Part model, mm, in its own coordinate system. A direction names the side the tool comes from. Give positions to 0.01 mm unless a question says otherwise; leave off trailing zeros. Order: outer loops, then holes, each group sorted by start corner. A loop starts at its lowest first (then second) coordinate and runs counter-clockwise, first axis right, second up. Notation, with made-up numbers: (-13.75, -32) - (16.25, -32) arc R22 ccw to (16.25, 1) - close; hole circle Ø3 at (-16.75, 9). An arc over 180 degrees is marked (long way). One line per item, written item: value.
```python
from build123d import *

# Parameters (mm, degrees)
MODEL_R                 = 1.7
MODEL_R_2               = 1.600279216
SALIENTE_EXTRUIR1_DEPTH = 3


with BuildPart() as part:
    # Model → Saliente-Extruir1 (new body)
    with BuildSketch(Plane.XY):
        with BuildLine():
            Line((74.679802956, 300.758040435), (5.677398721, 300.758040435))
            ThreePointArc((5.677398721, 300.758040435), (4.61673855, 300.318700606), (4.177398721, 299.258040435))
            Line((4.177398721, 299.258040435), (4.177398721, 221.253430577))
            ThreePointArc((4.177398721, 221.253430577), (4.61673855, 220.192770405), (5.677398721, 219.753430577))
            Line((5.677398721, 219.753430577), (28.17721751, 219.753430577))
            ThreePointArc((28.17721751, 219.753430577), (28.884324291, 220.046323796), (29.17721751, 220.753430577))
            Line((29.17721751, 220.753430577), (29.17721751, 227.730037779))
            ThreePointArc((29.17721751, 227.730037779), (28.884324291, 228.43714456), (28.17721751, 228.730037779))
            Line((28.17721751, 228.730037779), (7.17721751, 228.730037779))
            ThreePointArc((7.17721751, 228.730037779), (6.470110728, 229.022930998), (6.17721751, 229.730037779))
            Line((6.17721751, 229.730037779), (6.17721751, 291.370238846))
            ThreePointArc((6.17721751, 291.370238846), (6.470110728, 292.077345627), (7.17721751, 292.370238846))
            Line((7.17721751, 292.370238846), (19.67721751, 292.370238846))
            ThreePointArc((19.67721751, 292.370238846), (20.384324291, 292.663132064), (20.67721751, 293.370238846))
            Line((20.67721751, 293.370238846), (20.67721751, 298.097066693))
            ThreePointArc((20.67721751, 298.097066693), (20.970110728, 298.804173474), (21.67721751, 299.097066693))
            Line((21.67721751, 299.097066693), (58.179621744, 299.097066693))
            ThreePointArc((58.179621744, 299.097066693), (58.886728525, 298.804173474), (59.179621744, 298.097066693))
            Line((59.179621744, 298.097066693), (59.179621744, 294.260238845))
            ThreePointArc((59.179621744, 294.260238845), (59.472514963, 293.553132064), (60.179621744, 293.260238845))
            Line((60.179621744, 293.260238845), (73.179621744, 293.260238845))
            ThreePointArc((73.179621744, 293.260238845), (73.886728525, 292.967345627), (74.179621744, 292.260238845))
            Line((74.179621744, 292.260238845), (74.179621744, 227.755628988))
            ThreePointArc((74.179621744, 227.755628988), (73.886728525, 227.048522207), (73.179621744, 226.755628988))
            Line((73.179621744, 226.755628988), (56.179621744, 226.755628988))
            ThreePointArc((56.179621744, 226.755628988), (55.472514963, 226.462735769), (55.179621744, 225.755628988))
            Line((55.179621744, 225.755628988), (55.179621744, 220.753430577))
            ThreePointArc((55.179621744, 220.753430577), (55.472514963, 220.046323796), (56.179621744, 219.753430577))
            Line((56.179621744, 219.753430577), (74.679802956, 219.753430577))
            ThreePointArc((74.679802956, 219.753430577), (75.740463127, 220.192770405), (76.179802956, 221.253430577))
            Line((76.179802956, 221.253430577), (76.179802956, 299.258040435))
            ThreePointArc((76.179802956, 299.258040435), (75.740463127, 300.318700606), (74.679802956, 300.758040435))
        make_face()
        with Locations((17.676729717, 224.253096075)):
            Circle(MODEL_R, mode=Mode.SUBTRACT)
        with Locations((62.680137458, 224.253096075)):
            Circle(MODEL_R, mode=Mode.SUBTRACT)
        with Locations((8.677064219, 224.253096075)):
            Circle(MODEL_R_2, mode=Mode.SUBTRACT)
        with Locations((71.679802956, 224.253096075)):
            Circle(MODEL_R_2, mode=Mode.SUBTRACT)
        with Locations((17.676729717, 296.258040435)):
            Circle(MODEL_R, mode=Mode.SUBTRACT)
        with Locations((62.680137458, 296.258040435)):
            Circle(MODEL_R, mode=Mode.SUBTRACT)
        with Locations((71.679802956, 296.258040435)):
            Circle(MODEL_R_2, mode=Mode.SUBTRACT)
        with Locations((8.677064219, 296.258040435)):
            Circle(MODEL_R_2, mode=Mode.SUBTRACT)
    extrude(amount=SALIENTE_EXTRUIR1_DEPTH)


solid = part.part
```
1) Which spindle directions (+Z, -Z, +X, -X, +Y, -Y) get a long thin tool onto all of the face, cutting with end or side? Do faces 1 (the face through (18, 228.73, 1)), 2 (the face through (76.18, 260, 1)), 3 (the face through (55.18, 223, 1)). Say none if no direction does.
Answer:
face 1: +Z, -Z
face 2: +Z, -Z, +X, +Y, -Y
face 3: +Z, -Z, -Y
2) Slice it at A-A on x = 67.5. Write the cut outline in (y, z).
Answer:
outline: (219.75, 0) - (226.76, 0) - (226.76, 3) - (219.75, 3) - close; (293.26, 0) - (300.76, 0) - (300.76, 3) - (293.26, 3) - close
3) Slice it at C-C on x = 35. Write the cut outline in (y, z).
Answer:
outline: (299.1, 0) - (300.76, 0) - (300.76, 3) - (299.1, 3) - close
4) Slice it at B-B on y = 271. Write the cut outline in (x, z), then the cut area to 3 significant figures.
Answer:
outline: (4.18, 0) - (6.18, 0) - (6.18, 3) - (4.18, 3) - close; (74.18, 0) - (76.18, 0) - (76.18, 3) - (74.18, 3) - close
area: 12.0 mm2
5) Wall check: line 1 along X through (y, z) = (224.5, 1.15); line 2 along X through (y, z) = (270, 0.2); line 3 along Y through (x, z) = (26, 2.4). Give the ranges that are in metal, low to high. Write a range as [from, to].
Answer:
line 1: x = [4.18, 7.1], [10.26, 15.99], [19.36, 29.18], [55.18, 61], [64.36, 70.1], [73.26, 76.18]
line 2: x = [4.18, 6.18], [74.18, 76.18]
line 3: y = [219.75, 228.73], [299.1, 300.76]
6) Slice it at D-D on z = 1.3. Count the separate pieces of the cut face and the enclosed holes in it, then the cut area to 3 significant figures.
Answer:
separate pieces: 1
enclosed holes: 8
area: 891 mm2
7) Two-plate mould, pull along X, no slides. Class faces 4 (the face through (5, 260, 3)), 5 (the face through (61.33, 223.22, 1.48)), 6 (the face through (4.177, 261, 1)): pulls with the +X half, pulls with the -X half, needs draft (parallel to the pull), parting line crosses it, or undercut.
Answer:
face 4: needs draft
face 5: undercut
face 6: pulls with the -X half
8) Drop a flat-ended pin along its axis: P1, Ø4, axis at x = 8.68, y = 296.26, coming from the +Z side. Give the stop position or say it passes through.
Answer:
P1: stops at z = 3
